from build123d import *

# Parameters (mm, degrees)
F1_DEPTH = 46.736


with BuildPart() as f1:
    # F0 (on Right) → F1 (new body)
    with BuildSketch(Plane.YZ):
        with BuildLine():
            Line((-10.631341, 9.623196), (-10.631341, 0))
            Line((-10.631341, 0), (-59.388869, 0))
            Line((-59.388869, 0), (-59.388869, -29.602783))
            Line((-59.388869, -29.602783), (-44.175051, -29.602783))
            ThreePointArc((-44.175051, -29.602783), (-30.15268, -16.245136), (-16.13031, -29.602783))
            Line((-16.13031, -29.602783), (13.197524, -29.602783))
            ThreePointArc((13.197524, -29.602783), (28.961235, -17.830947), (44.724945, -29.602783))
            Line((44.724945, -29.602783), (63.604742, -29.602783))
            Line((63.604742, -29.602783), (63.604742, -10.356392))
            ThreePointArc((63.604742, -10.356392), (50.969791, -2.999156), (36.659796, 0))
            ThreePointArc((36.659796, 0), (25.687596, 6.901607), (13.014226, 9.623196))
            Line((13.014226, 9.623196), (-10.631341, 9.623196))
        make_face()
    extrude(amount=F1_DEPTH)


solid = f1.part
For this review, take the finished solid that the model builds, in its own axes (mm). A direction names the side the tool comes from. Round coordinates to 2 decimals unless told otherwise and drop trailing zeros. Write each loop counter-clockwise with the first axis right and the second up, starting at its lowest first coordinate (ties: lowest second). Pieces come first, ordered by that corner, then holes. Notation, with made-up numbers: (-10, 67) - (47, 67) arc R30 cw to (47, 91) - close; hole circle Ø10 at (-37, 66). An arc over 180 degrees is marked (long way). Use a Markdown table: item, result.
Q1. We need section C-C (y = -50). Give the boundary of the cut face in (x, z), plus the area to 3 significant figures.
Derived:
| item | result |
|---|---|
| outline | (0, -29.6) - (46.74, -29.6) - (46.74, 0) - (0, 0) - close |
| area | 1,380 mm2 |
Q2. Wall thickness on line 1 along Y through (x, z) = (22, -25.5); line 2 along Y through (x, z) = (35.5, -19.5); line 3 along Z through (x, y) = (4, -53): over which ranges is each line inside the solid? List them lowest first.
Derived:
| item | result |
|---|---|
| line 1 | y = -59.39 to -43.35, -16.95 to 15.06, 42.87 to 63.6 |
| line 2 | y = -59.39 to -39.14, -21.16 to 21.74, 36.18 to 63.6 |
| line 3 | z = -29.6 to 0 |
Q3. We need section D-D (z = 2). Give the boundary of the cut face in (x, y), plus the area to 3 significant figures.
Derived:
| item | result |
|---|---|
| outline | (0, -10.63) - (46.74, -10.63) - (46.74, 34.26) - (0, 34.26) - close |
| area | 2,100 mm2 |
Q4. The part is to be moulded in two halves that separate along Y. For faces 1 (the cylindrical face through (23.04, 25.86, 6.83)), 2 (the cylindrical face through (23.041, 28.666, -17.834)), 3 (the flat face through (23, 1, 9.623)), say which applies: pulls with the +Y half, pulls with the -Y half, needs draft (parallel to the pull), parting line crosses it, or undercut.
Derived:
| item | result |
|---|---|
| face 1 | pulls with the +Y half |
| face 2 | undercut |
| face 3 | needs draft |
Q5. We need section A-A (z = -23.5). Give the boundary of the cut face in (x, y).
Derived:
| item | result |
|---|---|
| outline | (0, -59.39) - (46.74, -59.39) - (46.74, -42.44) - (0, -42.44) - close; (0, -17.86) - (46.74, -17.86) - (46.74, 16.54) - (0, 16.54) - close; (0, 41.38) - (46.74, 41.38) - (46.74, 63.6) - (0, 63.6) - close |
Q6. Machinability: for faces 4 (the flat face through (23, -35, 0)), 5 (the flat face through (23, -2, -29.603)), which of the approach directions +Z, -Z, +X, -X, +Y, -Y give a long, thin tool a straight path to every point of the face, cutting with its end or side? Answer none if there is none.
Derived:
| item | result |
|---|---|
| face 4 | +Z, +X, -X, -Y |
| face 5 | -Z, +X, -X, +Y, -Y |
Q7. We need section B-B (x = 32.5). Give the boundary of the cut face in (y, z).
Derived:
| item | result |
|---|---|
| outline | (-59.39, -29.6) - (-44.18, -29.6) arc R14.04 cw to (-16.13, -29.6) - (13.2, -29.6) arc R16.44 cw to (44.72, -29.6) - (63.6, -29.6) - (63.6, -10.36) arc R45.79 ccw to (36.66, 0) arc R37.23 ccw to (13.01, 9.62) - (-10.63, 9.62) - (-10.63, 0) - (-59.39, 0) - close |
Q8. Clearance check with flat-ended pins moving along their axes: pin 1 (5 mm diameter, centred on x = 20, z = 6.5, fed in from -Y); pin 2 (1 mm diameter, centred on x = 16, y = -41.5, fed in from +Z); pin 3 (1.5 mm diameter, centred on x = 35.5, y = -40, fed in from -Z). State where each tip first meets the part, or that it passes through.
Derived:
| item | result |
|---|---|
| pin 1 | stops at y = -10.63 |
| pin 2 | stops at z = 0 |
| pin 3 | stops at z = -21.08 |
